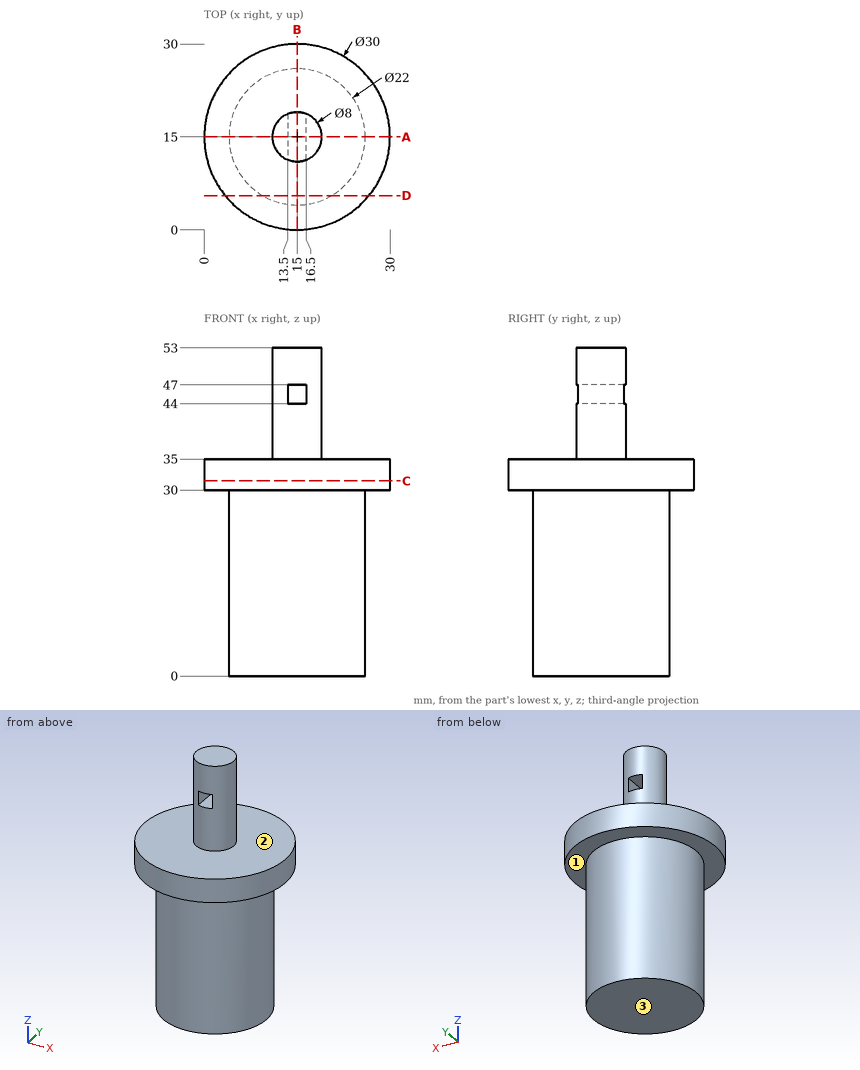
Print and shaded views of the part. All mm, measured from the part's lowest x, y and z. A direction names the side the tool comes from. Coordinates: 2 decimals unless noted, no trailing zeros. Loops run counter-clockwise (first coordinate to the right, second up) from the corner with the lowest first, then second, coordinate; pieces in that order, holes last. Notation, with made-up numbers: (75, 17.25) -> (121, 17.25) arc R28 cw to (121, 48.25) -> close; hole circle Ø3 at (45, 87.25). An arc over 180 degrees is marked (long way). Use a Markdown table: item, result. Add a question column.
Item 1: Probe probe 1 along Z at (x, y) = (17.75, 2.25); probe 2 along X at (y, z) = (18.5, 45); probe 3 along Z at (x, y) = (18.25, 10.5). List the from-to ranges inside material, lowest first.
Item 2: Band-saw the part on B-B on x = 15. Write the cut outline in (y, z), plus the area to 3 significant figures.
Item 3: Band-saw the part on A-A on y = 15. Write the cut outline in (x, z), plus the area to 3 significant figures.
Item 4: Band-saw the part on C-C on z = 31.5. Write the cut outline in (x, y).
Item 5: Band-saw the part on D-D on y = 5.5. Write the cut outline in (x, z), plus the area to 3 significant figures.
Item 6: Flat gauge pins, fed straight in: P1, Ø3, axis at y = 8.5, z = 7.5, coming from the +X side; P2, Ø0.9, axis at y = 16.5, z = 46, coming from the -X side; P3, Ø1.5, axis at y = 6.5, z = 25, coming from the +X side. Where does each tip first touch, or does it go through?
Item 7: Which spindle directions (+Z, -Z, +X, -X, +Y, -Y) get a long thin tool onto all of the face, cutting with end or side? Do the marked faces 1, 2 and 3. Say none if no direction does.
Geometry says:
| question | item | result |
|---|---|---|
| 1 | probe 1 | 30 to 35 |
| 1 | probe 2 | 13.06 to 13.5, 16.5 to 16.94 |
| 1 | probe 3 | 0 to 35 |
| 2 | outline | (0, 30) -> (4, 30) -> (4, 0) -> (26, 0) -> (26, 30) -> (30, 30) -> (30, 35) -> (19, 35) -> (19, 44) -> (11, 44) -> (11, 35) -> (0, 35) -> close; (11, 47) -> (19, 47) -> (19, 53) -> (11, 53) -> close |
| 2 | area | 930 mm² |
| 3 | outline | (0, 30) -> (4, 30) -> (4, 0) -> (26, 0) -> (26, 30) -> (30, 30) -> (30, 35) -> (19, 35) -> (19, 53) -> (11, 53) -> (11, 35) -> (0, 35) -> close; hole (13.5, 44) -> (16.5, 44) -> (16.5, 47) -> (13.5, 47) -> close |
| 3 | area | 945 mm² |
| 4 | outline | circle Ø30 at (15, 15) |
| 5 | outline | (3.39, 30) -> (9.45, 30) -> (9.45, 0) -> (20.55, 0) -> (20.55, 30) -> (26.61, 30) -> (26.61, 35) -> (3.39, 35) -> close |
| 5 | area | 449 mm² |
| 6 | P1 | x = 24.8 |
| 6 | P2 | x = 11.14 |
| 6 | P3 | x = 22.81 |
| 7 | face 1 | -Z |
| 7 | face 2 | +Z |
| 7 | face 3 | -Z, +X, -X, +Y, -Y |
